Input: dimensioned drawing with shaded views. Units: mm. Origin: part minimum x, y, z. A direction names the side the tool comes from. Round coordinates to 2 decimals unless told otherwise and drop trailing zeros. Loops run counter-clockwise (first coordinate to the right, second up) from the corner with the lowest first, then second, coordinate; pieces in that order, holes last. Notation, with made-up numbers: M 52,-9 L 106,-9 A8 ccw 106,-1 Z; hole C -6,25 d7. An arc over 180 degrees is marked long. Return JSON: item names as keys, results as strings.
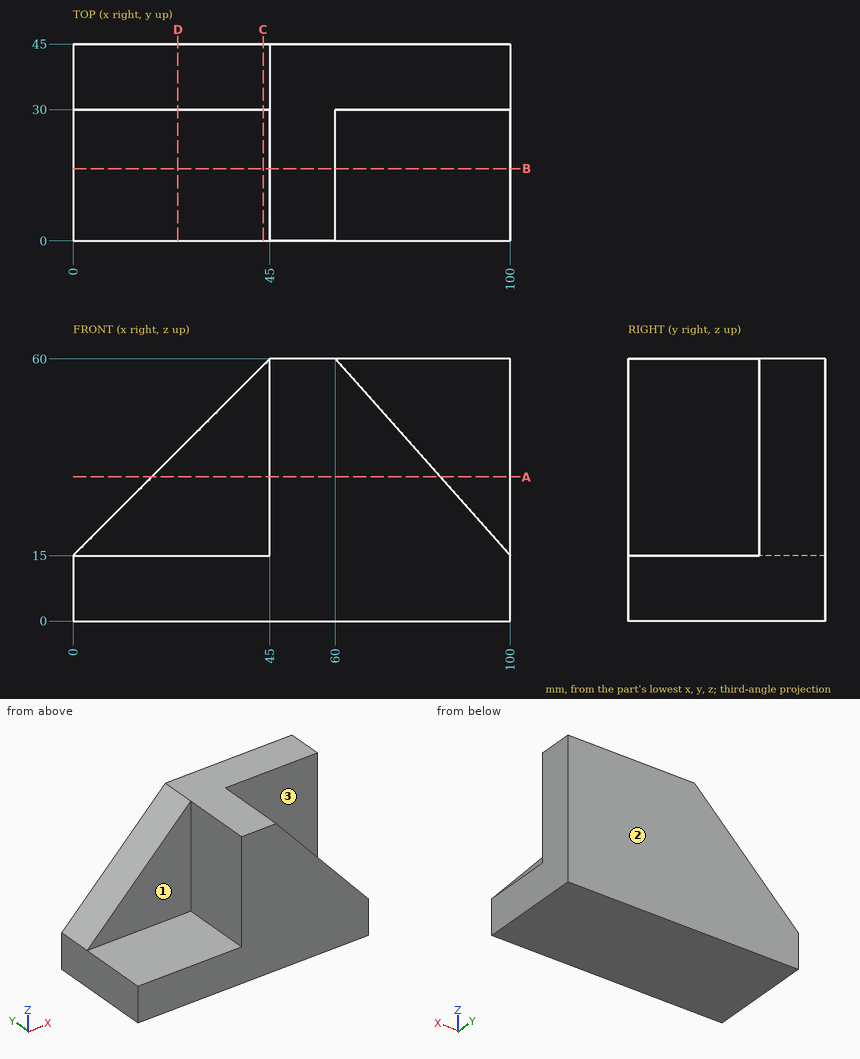
Q1. Section query A-A (z = 33). Output: boundary loops of the cut face in (x, y).
Determined:
{"outline": "M 18,30 L 45,30 L 45,0 L 84,0 L 84,30 L 100,30 L 100,45 L 18,45 Z"}
Q2. Material intervals for L1, parallel to Z at x = 7, y = 18; L2, parallel to Y at x = 94, z = 32; L3, parallel to Z at x = 96, y = 9.5, sorted ascending.
Determined:
{"L1": "z = 0 to 15", "L2": "y = 30 to 45", "L3": "z = 0 to 19.5"}
Q3. Pin query (flat end, axial travel): pin 1 (22.5 mm diameter, centred on x = 27, z = 41, fed in from -Y). Return the tip coordinate at first contact, or that it passes through.
Determined:
{"pin 1": "stops at y = 30"}
Q4. Reachability of the marked faces 1, 2 and 3 from +Z, -Z, +X, -X, +Y, -Y: full face, straight path, thin tool, end or side. Return the list, or none.
Determined:
{"face 1": "+Z, -X, -Y", "face 2": "+Z, -Z, +X, -X, +Y", "face 3": "+Z, +X, -Y"}
Q5. Section query D-D (x = 24). Output: boundary loops of the cut face in (y, z), plus the area to 4 significant figures.
Determined:
{"outline": "M 0,0 L 45,0 L 45,39 L 30,39 L 30,15 L 0,15 Z", "area": "1,035 mm^2"}
Q6. Section query B-B (y = 16.5). Output: boundary loops of the cut face in (x, z).
Determined:
{"outline": "M 0,0 L 100,0 L 100,15 L 60,60 L 45,60 L 45,15 L 0,15 Z"}
Q7. Section query C-C (x = 43.5). Output: boundary loops of the cut face in (y, z), plus the area to 3 significant figures.
Determined:
{"outline": "M 0,0 L 45,0 L 45,58.5 L 30,58.5 L 30,15 L 0,15 Z", "area": "1,330 mm^2"}
